from build123d import *

# Parameters (mm, degrees)
BOSS_EXTRUDE1_DEPTH              = 19.05
F_1_8_0_125_DIAMETER_HOLE1_D     = 3.175
F_1_8_0_125_DIAMETER_HOLE1_DEPTH = 11.1252
F_1_8_0_125_DIAMETER_HOLE1_TIP   = 0.953866233


with BuildPart() as part:
    # Sketch1 → Boss-Extrude1 (new body)
    with BuildSketch(Plane(origin=(0, 0, 0), x_dir=(1, 0, 0), z_dir=(0, 1, 0))):
        with BuildLine():
            Line((-99.020583087, -242.427582229), (-99.020583087, -374.65))
            ThreePointArc((-99.020583087, -374.65), (-89.495583087, -384.175), (-79.970583087, -374.65))
            Line((-79.970583087, -374.65), (-79.970583087, -245.266880288))
            ThreePointArc((-79.970583087, -245.266880288), (-78.028039526, -219.05629054), (-72.242855135, -193.418425341))
            Line((-72.242855135, -193.418425341), (-69.161727013, -183.311770075))
            ThreePointArc((-69.161727013, -183.311770075), (-36.664014716, -108.894116093), (12.050429612, -43.924958467))
            ThreePointArc((12.050429612, -43.924958467), (12.501856954, -40.160483954), (9.02530478, -38.647658789))
            ThreePointArc((9.02530478, -38.647658789), (-15.385960803, -36.583737732), (-33.934614128, -20.580078236))
            ThreePointArc((-33.934614128, -20.580078236), (-37.044039814, -19.076108136), (-39.686388117, -21.300619228))
            Line((-39.686388117, -21.300619228), (-91.292855135, -190.579127282))
            ThreePointArc((-91.292855135, -190.579127282), (-97.078039526, -216.216992482), (-99.020583087, -242.427582229))
        make_face()
    extrude(amount=BOSS_EXTRUDE1_DEPTH)

    # 1/8 (0.125) Diameter Hole1
    with Locations(Plane(origin=(0, 0, 0), x_dir=(-1, 0, 0), z_dir=(0, -1, 0))):
        with Locations((89.495583087, -358.775), (31.192579134, -50.114011233), (87.553039526, -217.636641511)):
            Hole(F_1_8_0_125_DIAMETER_HOLE1_D / 2, depth=F_1_8_0_125_DIAMETER_HOLE1_DEPTH)
            with Locations((0, 0, -(F_1_8_0_125_DIAMETER_HOLE1_DEPTH + F_1_8_0_125_DIAMETER_HOLE1_TIP / 2))):  # 118° drill point
                Cone(0, F_1_8_0_125_DIAMETER_HOLE1_D / 2, F_1_8_0_125_DIAMETER_HOLE1_TIP, mode=Mode.SUBTRACT)


solid = part.part
Part model, mm, in its own coordinate system. A direction names the side the tool comes from. Coordinates: 2 decimals unless noted, no trailing zeros. Loops run counter-clockwise (first coordinate to the right, second up) from the corner with the lowest first, then second, coordinate; pieces in that order, holes last. Notation, with made-up numbers: (-21.5, 72) - (18.5, 72) arc R25 cw to (18.5, 102) - close; hole circle Ø3 at (74, 35.25). An arc over 180 degrees is marked (long way). Write each question's results on one line, items separated by ' | '. Start each with the question number.
Q1. Drop flat-ended pins along their axis: pin 1 Ø6 at (y, z) = (6.5, 210.5) entering from -X; pin 2 Ø1.5 at (y, z) = (2.5, 97.5) entering from +X; pin 3 Ø3 at (y, z) = (15.5, 130) entering from +X. Give the stop position or say it passes through.
Q2. Slice it at C-C on x = -2. Give the cut face in (y, z).
Q3. Which spindle directions (+Z, -Z, +X, -X, +Y, -Y) get a long thin tool onto all of the face, cutting with end or side? Do faces 5 (the flat face through (-79.971, 9, 311)), 6 (the flat face through (-65.128, 9.392, 104.755)). Say none if no direction does.
Q4. Two-plate mould, pull along X, no slides. Class faces 1 (the cylindrical face through (-36.99, 9.39, 19.07)), 2 (the cylindrical face through (-37.236, 9.392, 109.88)), 3 (the cylindrical face through (-15.06, 9.39, 36.72)), 4 (the flat face through (-99.021, 9, 308)): +X half, -X half, draft (parallel to the pull), parting line (faces both ways), or undercut.
Q5. Slice it at A-A on y = 6. Give the number of separate pieces and of enclosed holes in the cut face, and give its area (3 significant figures).
Q6. Slice it at B-B on z = 281.5. Give the cut face in (x, y), and give its area (3 significant figures).
Q7. Probe line 1 along X through (y, z) = (1, 308); line 2 along X through (y, z) = (13.5, 54.5); line 3 along Z through (x, y) = (2.5, 11) (3 decimals). List the from-to ranges inside material, lowest first.
Answer:
1) pin 1: stops at x = -96.65 | pin 2: stops at x = -29.26 | pin 3: stops at x = -47.27
2) outline: (0, 39.64) - (19.05, 39.64) - (19.05, 59.65) - (0, 59.65) - close
3) face 5: +Z, +X, +Y, -Y | face 6: -Z, -X, +Y, -Y
4) face 1: parting line | face 2: +X half | face 3: undercut | face 4: -X half
5) separate pieces: 1 | enclosed holes: 3 | area: 8,870 mm2
6) outline: (-99.02, 0) - (-79.97, 0) - (-79.97, 19.05) - (-99.02, 19.05) - close | area: 363 mm2
7) line 1: x = -99.02 to -79.97 | line 2: x = -49.81 to 2.42 | line 3: z = 39.609 to 54.405
